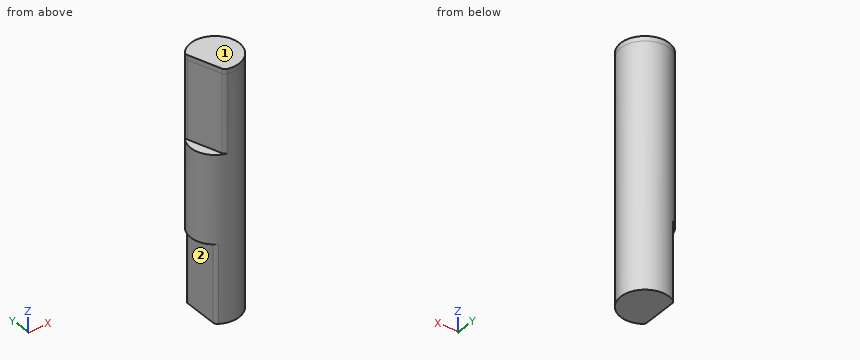
from build123d import *
from build123d.topology import SkipClean

# Parameters (mm, degrees)
SKETCH1_R           = 4.98
BOSS_EXTRUDE1_DEPTH = 50
CUT_EXTRUDE1_DEPTH  = 16
CUT_EXTRUDE2_START  = -16
CUT_EXTRUDE2_DEPTH  = 16
FILLET1_R           = 1
BOSS_EXTRUDE2_START = 1
BOSS_EXTRUDE2_DEPTH = 1


with BuildPart() as part:
    # Sketch1 → Boss-Extrude1 (new body)
    with BuildSketch(Plane.XY):
        Circle(SKETCH1_R)
    extrude(amount=BOSS_EXTRUDE1_DEPTH)

    # Sketch2 → Cut-Extrude1 (cut)
    with BuildSketch(Plane(origin=(0, 0, 0), x_dir=(-1, 0, 0), z_dir=(0, 0, -1))):
        Polygon((3, 37.964295833), (3, 3.974971698), (3, -3.974971698), (3, -37.964295833), (70.97864827, -37.964295833), (70.97864827, 37.964295833), align=None)
    extrude(amount=-CUT_EXTRUDE1_DEPTH, mode=Mode.SUBTRACT)

    # Sketch3 → Cut-Extrude2 (cut)
    with BuildSketch(Plane.XY.offset(50).offset(CUT_EXTRUDE2_START)):
        with BuildLine():
            Line((-1.570261684, -4.725957918), (-4.114243571, 2.805957918))
            ThreePointArc((-4.114243571, 2.805957918), (-4.718139362, -1.5936), (-1.570261684, -4.725957918))
        make_face()
    extrude(amount=CUT_EXTRUDE2_DEPTH, mode=Mode.SUBTRACT)

    # Fillet1
    fillet1_edges = [part.edges().sort_by_distance(p)[0] for p in [
        (-3, 3.974971698, 8),
        (-3, -3.974971698, 8),
        (-4.114243571, 2.805957918, 42),
        (-1.570261684, -4.725957918, 42),
    ]]
    fillet(fillet1_edges, radius=FILLET1_R)

    # Sketch4 → Boss-Extrude2 (add)
    with SkipClean():  # the faces are left unmerged after this step: merging them gives an invalid solid
        with BuildSketch(Plane.XY.offset(50).offset(BOSS_EXTRUDE2_START)):
            with BuildLine():
                Line((-3.943368861, 2.300052613), (-1.741136394, -4.220052613))
                ThreePointArc((-1.741136394, -4.220052613), (-1.455295916, -4.649929795), (-0.993145699, -4.87996533))
                ThreePointArc((-0.993145699, -4.87996533), (4.718139362, 1.5936), (-3.748702906, 3.27835729))
                ThreePointArc((-3.748702906, 3.27835729), (-3.97672335, 2.81520953), (-3.943368861, 2.300052613))
            make_face()
        extrude(amount=-BOSS_EXTRUDE2_DEPTH)


solid = part.part
Here's how the part is built. I have some questions about the finished solid (model axes, mm). Face numbers are marked on the shaded views. A direction names the side the tool comes from. Coordinates: 2 decimals unless noted, no trailing zeros. Order: outer loops, then holes, each group sorted by start corner. A loop starts at its lowest first (then second) coordinate and runs counter-clockwise, first axis right, second up.
Item 1: If we section it at B-B on z = 14.5: List the corners of the cut face in (x, y) for me.
Result sheet:
outline: (-3, -3.44) arc R1 ccw to (-2.5, -4.31) arc R4.98 ccw (long way) to (-2.5, 4.31) arc R1 ccw to (-3, 3.44) - close
Item 2: If we section it at C-C on x = 3.25: List the corners of the cut face in (y, z) for me, plus the area to 3 significant figures.
Result sheet:
outline: (-3.77, 0) - (3.77, 0) - (3.77, 51) - (-3.77, 51) - close
area: 385 mm2
Item 3: For P1, Ø2, axis at y = 0, z = 42.5, coming from the -X side; P2, Ø1.5, axis at y = -2.5, z = 18.5, coming from the +X side; P3, Ø4, axis at x = -3.5, y = -1.5, coming from the -Z side, each with a flat end and sliding along its axis, tell me the tip position at first contact or that it passes through.
Result sheet:
P1: stops at x = -3.5
P2: stops at x = 4.66
P3: stops at z = 0
Item 4: For the marked faces 1 and 2, which set-ups out of +Z, -Z, +X, -X, +Y, -Y let a thin tool reach every point of the face, with its end or its side?
Result sheet:
face 1: +Z, +X, -X, +Y, -Y
face 2: -Z, -X, +Y, -Y
Item 5: I need wall thicknesses on line 1 (Z direction, x = -3.25, y = -0.25); line 2 (X direction, y = -0.25, z = 5); line 3 (Z direction, x = -3.5, y = 2.5). Which ranges of each line are inside material? Lowest first, please.
Result sheet:
line 1: z = 16 to 34
line 2: x = -3 to 4.97
line 3: z = 16 to 51
Item 6: If we section it at A-A on y = 0: List the corners of the cut face in (x, z) for me, plus the area to 3 significant figures.
Result sheet:
outline: (-4.98, 16) - (-3, 16) - (-3, 0) - (4.98, 0) - (4.98, 51) - (-3.17, 51) - (-3.17, 34) - (-4.98, 34) - close
area: 445 mm2
